Verification items for the finished model (mm, model axes). A direction names the side the tool comes from. Coordinates: 2 decimals unless noted, no trailing zeros. Order: outer loops, then holes, each group sorted by start corner. A loop starts at its lowest first (then second) coordinate and runs counter-clockwise, first axis right, second up. Notation, with made-up numbers: M 41.5,-23.75 L 86.5,-23.75 A23 ccw 86.5,5.25 Z; hole C -28.75,36.5 d8. An arc over 180 degrees is marked long. Answer as a JSON object with one key per item and string values. Group by question number.
(1) Cross-section at D-D (y = 66). Enter the section's corners in (x, z).
(2) Gauge pin test, flat end, axial feed: pin 1 Ø4 at (x, y) = (-9, 56.5) entering from +Z. Record the tip position at first contact, or that the pin passes through.
(3) Material ranges on line 1 (Y direction, x = -30, z = 1.85); line 2 (Z direction, x = -24, y = 26.5); line 3 (Y direction, x = -14, z = 1.5), recorded low to high.
(4) Access from +Z, -Z, +X, -X, +Y, -Y to the whole of each face (thin tool, end or side, straight path). Record for faces 1 (the face through (-40, 44, 2)), 2 (the face through (-22.5, 0.1, 14.9)).
(5) Cross-section at B-B (x = -10). Enter the section's corners in (y, z), plus the area to 3 significant figures.
(6) Cross-section at C-C (x = -20). Enter the section's corners in (y, z), plus the area to 3 significant figures.
(7) Cross-section at A-A (y = 40). Enter the section's corners in (x, z).
(8) Mould release check, pull along Y, two halves, no side actions. Record for faces 3 (the face through (-20, -20, 2)), 4 (the face through (-28.925, 61.686, 2.535)), 5 (the face through (-20, 36, 5)): released by +Y, released by -Y, zero draft, split by the parting line, or undercut.
from build123d import *

# Parameters (mm, degrees)
BOSS_EXTRUDE1_DEPTH = 5
SKETCH2_R           = 2.5
BOSS_EXTRUDE2_DEPTH = 20
SKETCH3_R           = 2
CUT_EXTRUDE1_DEPTH  = 50
SKETCH5_R           = 2
CUT_EXTRUDE2_DEPTH  = 50
LPATTERN1_COUNT     = 2
LPATTERN1_PITCH     = 20


with BuildPart() as part:
    # Sketch1 → Boss-Extrude1 (new body)
    with BuildSketch(Plane.XY):
        with BuildLine():
            Line((-40, 90), (0, 90))
            Line((0, 90), (0, 0))
            ThreePointArc((0, 0), (-20, -20), (-40, 0))
            Line((-40, 0), (-40, 90))
        make_face()
    extrude(amount=BOSS_EXTRUDE1_DEPTH)

    # Sketch2 → Boss-Extrude2 (add)
    with BuildSketch(Plane.XY.offset(5)):
        with Locations((-20, 0)):
            Circle(SKETCH2_R)
    extrude(amount=BOSS_EXTRUDE2_DEPTH)

    # Sketch3 → Cut-Extrude1 (cut)
    with BuildSketch(Plane.XY.offset(5)):
        with Locations((-30, 85)):
            Circle(SKETCH3_R)
        with Locations((-10, 85)):
            Circle(SKETCH3_R)
    cut_extrude1 = extrude(amount=-CUT_EXTRUDE1_DEPTH, mode=Mode.SUBTRACT)

    # Sketch5 → Cut-Extrude2 (cut)
    with BuildSketch(Plane.XY.offset(5)):
        with Locations((-30, 60)):
            Circle(SKETCH5_R)
        with Locations((-10, 60)):
            Circle(SKETCH5_R)
    cut_extrude2 = extrude(amount=-CUT_EXTRUDE2_DEPTH, mode=Mode.SUBTRACT)

    # LPattern1: Cut-Extrude1, Cut-Extrude2 ×2
    with Locations(*[(0, -i * LPATTERN1_PITCH, 0) for i in range(1, LPATTERN1_COUNT)]):
        add(cut_extrude1, mode=Mode.SUBTRACT)
        add(cut_extrude2, mode=Mode.SUBTRACT)


solid = part.part
Taken from the geometry:
{
 "1": {"outline": "M -40,0 L -31.73,0 L -31.73,5 L -40,5 Z; M -28.27,0 L -11.73,0 L -11.73,5 L -28.27,5 Z; M -8.27,0 L 0,0 L 0,5 L -8.27,5 Z"},
 "2": {"pin 1": "stops at z = 5"},
 "3": {"line 1": "y = -17.32 to 38, 42 to 58, 62 to 63, 67 to 83, 87 to 90", "line 2": "z = 0 to 5", "line 3": "y = -19.08 to 90"},
 "4": {"face 1": "+Z, -Z, -X, +Y, -Y", "face 2": "+Z"},
 "5": {"outline": "M -17.32,0 L 38,0 L 38,5 L -17.32,5 Z; M 42,0 L 58,0 L 58,5 L 42,5 Z; M 62,0 L 63,0 L 63,5 L 62,5 Z; M 67,0 L 83,0 L 83,5 L 67,5 Z; M 87,0 L 90,0 L 90,5 L 87,5 Z", "area": "457 mm²"},
 "6": {"outline": "M -20,0 L 90,0 L 90,5 L 2.5,5 L 2.5,25 L -2.5,25 L -2.5,5 L -20,5 Z", "area": "650 mm²"},
 "7": {"outline": "M -40,0 L -32,0 L -32,5 L -40,5 Z; M -28,0 L -12,0 L -12,5 L -28,5 Z; M -8,0 L 0,0 L 0,5 L -8,5 Z"},
 "8": {"face 3": "released by -Y", "face 4": "undercut", "face 5": "zero draft"}
}
